Could you check a few things on this model? Use its own coordinates, in mm. Face numbers are marked on the shaded views. A direction names the side the tool comes from. Round coordinates to 2 decimals unless told otherwise and drop trailing zeros. Loops run counter-clockwise (first coordinate to the right, second up) from the corner with the lowest first, then second, coordinate; pieces in that order, holes last. Notation, with made-up numbers: (58, 39) -> (89, 39) arc R6 ccw to (89, 43) -> close; hole circle Ø8 at (65, -6). An arc over 180 degrees is marked (long way). One line per item, written item: value.
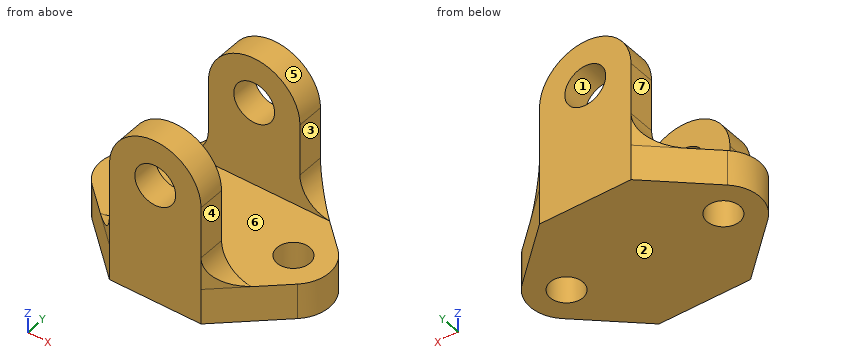
```python
from build123d import *

# Parameters (mm, degrees)
SKETCH1_W                      = 46.48
SKETCH1_H                      = 30.48
SKETCH1_R                      = 3.175
BOSS_EXTRUDE1_DEPTH            = 9.46
SKETCH2_W                      = 46.48
SKETCH2_H                      = 5.24
BOSS_EXTRUDE2_DEPTH            = 53
CUT_EXTRUDE1_REACH             = 70.364
SKETCH4_R                      = 3.96875
CUT_EXTRUDE1_DIRECTION_2_REACH = 70.364
CUT_EXTRUDE3_REACH             = 70.364
CUT_EXTRUDE3_DIRECTION_2_REACH = 70.364
CUT_EXTRUDE4_DEPTH             = 9.46
BOSS_EXTRUDE3_DEPTH            = 9.46
FILLET3_R                      = 6.35
CUT_EXTRUDE5_DEPTH             = 2.54


with BuildPart() as part:
    # Sketch1 → Boss-Extrude1 (new body)
    with BuildSketch(Plane.XY):
        Rectangle(SKETCH1_W, SKETCH1_H)
        with Locations((15.24, 0)):
            Circle(SKETCH1_R, mode=Mode.SUBTRACT)
        with Locations((-15.24, 0)):
            Circle(SKETCH1_R, mode=Mode.SUBTRACT)
    extrude(amount=BOSS_EXTRUDE1_DEPTH)

    # Sketch2 → Boss-Extrude2 (add)
    with BuildSketch(Plane.XY.offset(9.46)):
        with Locations((0, 12.62)):
            Rectangle(SKETCH2_W, SKETCH2_H)
        with Locations((0, -12.62)):
            Rectangle(SKETCH2_W, SKETCH2_H)
    extrude(amount=BOSS_EXTRUDE2_DEPTH)

    # Cut-Extrude1: up to this face of the body (flat: up to its plane)
    cut_extrude1_end = Plane(part.part.faces().sort_by_distance((0, -15.24, 31.23))[0])
    # Sketch4 → Cut-Extrude1 (cut, up to the picked face)
    with BuildSketch(Plane(origin=(0, 0, 0), x_dir=(1, 0, 0), z_dir=(0, 1, 0)), mode=Mode.PRIVATE) as cut_extrude1_sk1:
        with Locations(Location((0, -25.8481308, 0), (0, 0, 270))):
            Circle(SKETCH4_R)
    cut_extrude1_tool1 = split(extrude(cut_extrude1_sk1.sketch, amount=-CUT_EXTRUDE1_REACH, mode=Mode.PRIVATE), bisect_by=cut_extrude1_end, keep=Keep.BOTH, mode=Mode.PRIVATE)
    add(cut_extrude1_tool1.solids().sort_by(Axis((0, 0, 25.848131), (0, -1, 0)))[0], mode=Mode.SUBTRACT)

    # Cut-Extrude1 direction 2: up to this face of the body (flat: up to its plane)
    cut_extrude1_direction_2_end = Plane(part.part.faces().sort_by_distance((0, 15.24, 31.23))[0])
    # Sketch4 → Cut-Extrude1 direction 2 (cut, up to the picked face)
    with BuildSketch(Plane(origin=(0, 0, 0), x_dir=(1, 0, 0), z_dir=(0, 1, 0)), mode=Mode.PRIVATE) as cut_extrude1_direction_2_sk1:
        with Locations(Location((0, -25.8481308, 0), (0, 0, 270))):
            Circle(SKETCH4_R)
    cut_extrude1_direction_2_tool1 = split(extrude(cut_extrude1_direction_2_sk1.sketch, amount=CUT_EXTRUDE1_DIRECTION_2_REACH, mode=Mode.PRIVATE), bisect_by=cut_extrude1_direction_2_end, keep=Keep.BOTH, mode=Mode.PRIVATE)
    add(cut_extrude1_direction_2_tool1.solids().sort_by(Axis((0, 0, 25.848131), (0, 1, 0)))[0], mode=Mode.SUBTRACT)

    # Cut-Extrude3: up to this face of the body (flat: up to its plane)
    cut_extrude3_end = Plane(part.part.faces().sort_by_distance((0, -15.24, 31.323322986))[0])
    # Sketch6 → Cut-Extrude3 (cut, up to the picked face)
    with BuildSketch(Plane(origin=(0, 0, 0), x_dir=(1, 0, 0), z_dir=(0, 1, 0)), mode=Mode.PRIVATE) as cut_extrude3_sk1:
        with BuildLine():
            Line((-8.89, -25.8481308), (-8.89, -17.46))
            Line((-8.89, -17.46), (-8.89, -9.46))
            Line((-8.89, -9.46), (-16.89, -9.46))
            Line((-16.89, -9.46), (-23.24, -9.46))
            Line((-23.24, -9.46), (-23.24, -62.46))
            Line((-23.24, -62.46), (23.24, -62.46))
            Line((23.24, -62.46), (23.24, -9.46))
            Line((23.24, -9.46), (16.89, -9.46))
            Line((16.89, -9.46), (8.89, -9.46))
            Line((8.89, -9.46), (8.89, -17.46))
            Line((8.89, -17.46), (8.89, -25.8481308))
            ThreePointArc((8.89, -25.8481308), (0, -34.7381308), (-8.89, -25.8481308))
        make_face()
    cut_extrude3_tool1 = split(extrude(cut_extrude3_sk1.sketch, amount=-CUT_EXTRUDE3_REACH, mode=Mode.PRIVATE), bisect_by=cut_extrude3_end, keep=Keep.BOTH, mode=Mode.PRIVATE)
    add(cut_extrude3_tool1.solids().sort_by(Axis((0, 0, 38.948856), (0, -1, 0)))[0], mode=Mode.SUBTRACT)

    # Cut-Extrude3 direction 2: up to this face of the body (flat: up to its plane)
    cut_extrude3_direction_2_end = Plane(part.part.faces().sort_by_distance((0, 15.24, 31.323322986))[0])
    # Sketch6 → Cut-Extrude3 direction 2 (cut, up to the picked face)
    with BuildSketch(Plane(origin=(0, 0, 0), x_dir=(1, 0, 0), z_dir=(0, 1, 0)), mode=Mode.PRIVATE) as cut_extrude3_direction_2_sk1:
        with BuildLine():
            Line((-8.89, -25.8481308), (-8.89, -17.46))
            Line((-8.89, -17.46), (-8.89, -9.46))
            Line((-8.89, -9.46), (-16.89, -9.46))
            Line((-16.89, -9.46), (-23.24, -9.46))
            Line((-23.24, -9.46), (-23.24, -62.46))
            Line((-23.24, -62.46), (23.24, -62.46))
            Line((23.24, -62.46), (23.24, -9.46))
            Line((23.24, -9.46), (16.89, -9.46))
            Line((16.89, -9.46), (8.89, -9.46))
            Line((8.89, -9.46), (8.89, -17.46))
            Line((8.89, -17.46), (8.89, -25.8481308))
            ThreePointArc((8.89, -25.8481308), (0, -34.7381308), (-8.89, -25.8481308))
        make_face()
    cut_extrude3_direction_2_tool1 = split(extrude(cut_extrude3_direction_2_sk1.sketch, amount=CUT_EXTRUDE3_DIRECTION_2_REACH, mode=Mode.PRIVATE), bisect_by=cut_extrude3_direction_2_end, keep=Keep.BOTH, mode=Mode.PRIVATE)
    add(cut_extrude3_direction_2_tool1.solids().sort_by(Axis((0, 0, 38.948856), (0, 1, 0)))[0], mode=Mode.SUBTRACT)

    # Sketch7 → Cut-Extrude4 (cut)
    with BuildSketch(Plane.XY):
        with BuildLine():
            ThreePointArc((-15.24, -7), (-22.24, 0), (-15.24, 7))
            Line((-15.24, 7), (-8.89, 7))
            Line((-8.89, 7), (-8.89, 15.24))
            Line((-8.89, 15.24), (-23.24, 15.24))
            Line((-23.24, 15.24), (-23.24, -15.24))
            Line((-23.24, -15.24), (-8.89, -15.24))
            Line((-8.89, -15.24), (-8.89, -7))
            Line((-8.89, -7), (-15.24, -7))
        make_face()
        with BuildLine():
            Line((8.89, 15.24), (8.89, 7))
            Line((8.89, 7), (15.24, 7))
            ThreePointArc((15.24, 7), (22.24, 0), (15.24, -7))
            Line((15.24, -7), (8.89, -7))
            Line((8.89, -7), (8.89, -15.24))
            Line((8.89, -15.24), (23.24, -15.24))
            Line((23.24, -15.24), (23.24, 15.24))
            Line((23.24, 15.24), (8.89, 15.24))
        make_face()
    extrude(amount=CUT_EXTRUDE4_DEPTH, mode=Mode.SUBTRACT)

    # Sketch8 → Boss-Extrude3 (add)
    with BuildSketch(Plane.XY):
        with BuildLine():
            Line((8.89, -15.24), (19.950515714, -5.177937978))
            ThreePointArc((19.950515714, -5.177937978), (17.765315243, -6.528612634), (15.24, -7))
            Line((15.24, -7), (8.89, -7))
            Line((8.89, -7), (8.89, -15.24))
        make_face()
        with BuildLine():
            ThreePointArc((-19.950515714, -5.177937978), (-17.765315243, -6.528612634), (-15.24, -7))
            Line((-15.24, -7), (-8.89, -7))
            Line((-8.89, -7), (-8.89, -15.24))
            Line((-8.89, -15.24), (-19.950515714, -5.177937978))
        make_face()
        with BuildLine():
            Line((8.89, 15.24), (19.950515714, 5.177937978))
            ThreePointArc((19.950515714, 5.177937978), (17.765315243, 6.528612634), (15.24, 7))
            Line((15.24, 7), (8.89, 7))
            Line((8.89, 7), (8.89, 15.24))
        make_face()
        with BuildLine():
            Line((-8.89, 15.24), (-19.950515714, 5.177937978))
            ThreePointArc((-19.950515714, 5.177937978), (-17.765315243, 6.528612634), (-15.24, 7))
            Line((-15.24, 7), (-8.89, 7))
            Line((-8.89, 7), (-8.89, 15.24))
        make_face()
    extrude(amount=BOSS_EXTRUDE3_DEPTH)

    # Fillet3
    # the kernel refuses this fillet: 6.35 mm, written as the material it adds along each edge
    with BuildSketch(Plane(origin=(8.89, -10, 9.46), x_dir=(0, 0, 1), z_dir=(0, -1, 0))) as fillet3_piece_1_section:
        with BuildLine():
            CenterArc((FILLET3_R, -FILLET3_R), FILLET3_R, 90, 90)
            Line((0, -FILLET3_R), (0, 0))
            Line((0, 0), (FILLET3_R, 0))
        make_face()
    fillet3_piece_1 = extrude(amount=5.24, mode=Mode.PRIVATE)
    fillet3_piece_1 = split(fillet3_piece_1, bisect_by=Plane(origin=(10.975439596, -13.342816984, 11.151175663), z_dir=(-0.6729308163346117, 0.7397054254412585, 0)), keep=Keep.TOP, mode=Mode.PRIVATE)
    add(fillet3_piece_1)
    with BuildSketch(Plane(origin=(-8.89, -10, 9.46), x_dir=(0, 0, 1), z_dir=(0, -1, 0))) as fillet3_piece_2_section:
        with BuildLine():
            CenterArc((FILLET3_R, FILLET3_R), FILLET3_R, 180, 90)
            Line((0, FILLET3_R), (0, 0))
            Line((0, 0), (FILLET3_R, 0))
        make_face()
    fillet3_piece_2 = extrude(amount=5.24, mode=Mode.PRIVATE)
    fillet3_piece_2 = split(fillet3_piece_2, bisect_by=Plane(origin=(-10.975439596, -13.342816984, 11.151175663), z_dir=(0.6729308163346114, 0.7397054254412588, 0)), keep=Keep.TOP, mode=Mode.PRIVATE)
    add(fillet3_piece_2)
    with BuildSketch(Plane(origin=(8.89, 10, 9.46), x_dir=(1, 0, 0), z_dir=(0, 1, 0))) as fillet3_piece_3_section:
        with BuildLine():
            CenterArc((FILLET3_R, -FILLET3_R), FILLET3_R, 90, 90)
            Line((0, -FILLET3_R), (0, 0))
            Line((0, 0), (FILLET3_R, 0))
        make_face()
    fillet3_piece_3 = extrude(amount=5.24, mode=Mode.PRIVATE)
    fillet3_piece_3 = split(fillet3_piece_3, bisect_by=Plane(origin=(10.975439596, 13.342816985, 11.151175663), z_dir=(-0.6729308163346115, -0.7397054254412587, 0)), keep=Keep.TOP, mode=Mode.PRIVATE)
    add(fillet3_piece_3)
    with BuildSketch(Plane(origin=(-8.89, 10, 9.46), x_dir=(-1, 0, 0), z_dir=(0, 1, 0))) as fillet3_piece_4_section:
        with BuildLine():
            CenterArc((FILLET3_R, FILLET3_R), FILLET3_R, 180, 90)
            Line((0, FILLET3_R), (0, 0))
            Line((0, 0), (FILLET3_R, 0))
        make_face()
    fillet3_piece_4 = extrude(amount=5.24, mode=Mode.PRIVATE)
    fillet3_piece_4 = split(fillet3_piece_4, bisect_by=Plane(origin=(-10.975439596, 13.342816985, 11.151175663), z_dir=(0.6729308163346117, -0.7397054254412585, 0)), keep=Keep.TOP, mode=Mode.PRIVATE)
    add(fillet3_piece_4)

    # Sketch10 → Cut-Extrude5 (cut)
    with BuildSketch(Plane.XY):
        with BuildLine():
            Line((-8.89, 15.24), (-19.950515714, 5.177937978))
            ThreePointArc((-19.950515714, 5.177937978), (-22.24, 0), (-19.950515714, -5.177937978))
            Line((-19.950515714, -5.177937978), (-8.89, -15.24))
            Line((-8.89, -15.24), (8.89, -15.24))
            Line((8.89, -15.24), (19.950515714, -5.177937978))
            ThreePointArc((19.950515714, -5.177937978), (22.24, 0), (19.950515714, 5.177937978))
            Line((19.950515714, 5.177937978), (8.89, 15.24))
            Line((8.89, 15.24), (-8.89, 15.24))
        make_face()
    extrude(amount=CUT_EXTRUDE5_DEPTH, mode=Mode.SUBTRACT)


solid = part.part
```
Item 1: I need wall thicknesses on line 1 (X direction, y = 0, z = 5.5) (3 decimals); line 2 (Y direction, x = 4.5, z = 17); line 3 (Z direction, x = 0, y = 13.3). Which ranges of each line are inside material? Lowest first, please. Write a range as from..to.
Output:
line 1: x = -22.24..-18.415, -12.065..12.065, 18.415..22.24
line 2: y = -15.24..-10, 10..15.24
line 3: z = 2.54..21.88, 29.82..34.74
Item 2: Will these pins go through, and if not, where does the flat tip stop? pin 1 Ø6 at (y, z) = (11.5, 20.5) entering from -X; pin 2 Ø5 at (y, z) = (9, 14.5) entering from +X; pin 3 Ø6 at (y, z) = (13.5, 20.5) entering from +X.
Output:
pin 1: stops at x = -8.89
pin 2: stops at x = 10.01
pin 3: stops at x = 8.89
Item 3: If we section it at C-C on y = 0: List the corners of the cut face in (x, z) for me (3 decimals), plus the area to 3 significant figures.
Output:
outline: (-22.24, 2.54) -> (-18.415, 2.54) -> (-18.415, 9.46) -> (-22.24, 9.46) -> close; (-12.065, 2.54) -> (12.065, 2.54) -> (12.065, 9.46) -> (-12.065, 9.46) -> close; (18.415, 2.54) -> (22.24, 2.54) -> (22.24, 9.46) -> (18.415, 9.46) -> close
area: 220 mm²
Item 4: For the marked faces 4, 5, 6 and 7, which set-ups out of +Z, -Z, +X, -X, +Y, -Y let a thin tool reach every point of the face, with its end or its side?
Output:
face 4: +Z, +X, +Y, -Y
face 5: +Z, +Y, -Y
face 6: +Z, +X, -X
face 7: +Z, -X, +Y, -Y
Item 5: If we section it at D-D on z = 23.5: List the corners of the cut face in (x, y) for me.
Output:
outline: (-8.89, -15.24) -> (-3.2, -15.24) -> (-3.2, -10) -> (-8.89, -10) -> close; (-8.89, 10) -> (-3.2, 10) -> (-3.2, 15.24) -> (-8.89, 15.24) -> close; (3.2, -15.24) -> (8.89, -15.24) -> (8.89, -10) -> (3.2, -10) -> close; (3.2, 10) -> (8.89, 10) -> (8.89, 15.24) -> (3.2, 15.24) -> close
Item 6: If we section it at B-B on z = 20: List the corners of the cut face in (x, y) for me.
Output:
outline: (-8.89, -15.24) -> (8.89, -15.24) -> (8.89, -10) -> (-8.89, -10) -> close; (-8.89, 10) -> (8.89, 10) -> (8.89, 15.24) -> (-8.89, 15.24) -> close
Item 7: If we section it at A-A on x = 0: List the corners of the cut face in (y, z) for me, plus the area to 3 significant figures.
Output:
outline: (-15.24, 2.54) -> (15.24, 2.54) -> (15.24, 21.88) -> (10, 21.88) -> (10, 9.46) -> (-10, 9.46) -> (-10, 21.88) -> (-15.24, 21.88) -> close; (-15.24, 29.82) -> (-10, 29.82) -> (-10, 34.74) -> (-15.24, 34.74) -> close; (10, 29.82) -> (15.24, 29.82) -> (15.24, 34.74) -> (10, 34.74) -> close
area: 393 mm²
Item 8: If we mould it in two halves opening along X, with no side actions, what happens to the marked faces 1, 2 and 3? For each: released by +X, released by -X, zero draft, split by the parting line, or undercut.
Output:
face 1: undercut
face 2: zero draft
face 3: released by +X
